from build123d import *

# Parameters (mm, degrees)
SKETCH1_W           = 40.5
SKETCH1_H           = 20
BOSS_EXTRUDE1_DEPTH = 41
SKETCH2_W           = 56.4
SKETCH2_H           = 20
SKETCH2_R           = 2.25
BOSS_EXTRUDE2_DEPTH = 3.5
SKETCH3_R           = 3
BOSS_EXTRUDE3_DEPTH = 6
SKETCH4_W           = 10
SKETCH4_H           = 3.5
BOSS_EXTRUDE4_DEPTH = 5
FILLET1_R           = 2
FILLET2_R           = 1
FILLET3_R           = 1


with BuildPart() as part:
    # Sketch1 → Boss-Extrude1 (new body)
    with BuildSketch(Plane(origin=(0, 0, 0), x_dir=(1, 0, 0), z_dir=(0, 1, 0))):
        Rectangle(SKETCH1_W, SKETCH1_H)
    extrude(amount=BOSS_EXTRUDE1_DEPTH)

    # Sketch2 → Boss-Extrude2 (add)
    with BuildSketch(Plane(origin=(0, 28, 0), x_dir=(-1, 0, 0), z_dir=(0, -1, 0))):
        Rectangle(SKETCH2_W, SKETCH2_H)
        with Locations(Location((-24, 5, 0), (0, 0, 90))):
            Circle(SKETCH2_R, mode=Mode.SUBTRACT)
        with Locations(Location((24, 5, 0), (0, 0, 90))):
            Circle(SKETCH2_R, mode=Mode.SUBTRACT)
        with Locations(Location((24, -5, 0), (0, 0, 90))):
            Circle(SKETCH2_R, mode=Mode.SUBTRACT)
        with Locations(Location((-24, -5, 0), (0, 0, 90))):
            Circle(SKETCH2_R, mode=Mode.SUBTRACT)
    extrude(amount=-BOSS_EXTRUDE2_DEPTH)

    # Sketch3 → Boss-Extrude3 (add)
    with BuildSketch(Plane(origin=(0, 41, 0), x_dir=(1, 0, 0), z_dir=(0, 1, 0))):
        with Locations(Location((-10.5, 0, 0), (0, 0, 270))):
            Circle(SKETCH3_R)
    extrude(amount=BOSS_EXTRUDE3_DEPTH)

    # Sketch4 → Boss-Extrude4 (add)
    with BuildSketch(Plane.ZY.offset(20.25)):
        with Locations((0, 5.25)):
            Rectangle(SKETCH4_W, SKETCH4_H)
    extrude(amount=BOSS_EXTRUDE4_DEPTH)

    # Fillet1
    fillet1_edges = [part.edges().sort_by_distance(p)[0] for p in [
        (28.2, 29.75, -10),
        (-28.2, 29.75, 10),
        (28.2, 29.75, 10),
        (-28.2, 29.75, -10),
    ]]
    fillet(fillet1_edges, radius=FILLET1_R)

    # Fillet2
    fillet2_edges = [part.edges().sort_by_distance(p)[0] for p in [
        (20.25, 14, 10),
        (-20.25, 14, 10),
        (-20.25, 14, -10),
        (20.25, 14, -10),
        (0, 0, 10),
        (-20.25, 0, 0),
        (0, 0, -10),
        (20.25, 0, 0),
        (-20.25, 36.25, 10),
        (-20.25, 36.25, -10),
    ]]
    fillet(fillet2_edges, radius=FILLET2_R)

    # Fillet3
    fillet3_edges = [part.edges().sort_by_distance(p)[0] for p in [
        (0.5, 41, 10),
        (-20.25, 41, 0),
        (-19.957106781, 41, 9.707106781),
        (-19.957106781, 41, -9.707106781),
        (20.25, 41, 0),
        (20.25, 36.25, 10),
        (20.25, 36.25, -10),
        (0.5, 41, -10),
    ]]
    fillet(fillet3_edges, radius=FILLET3_R)


solid = part.part
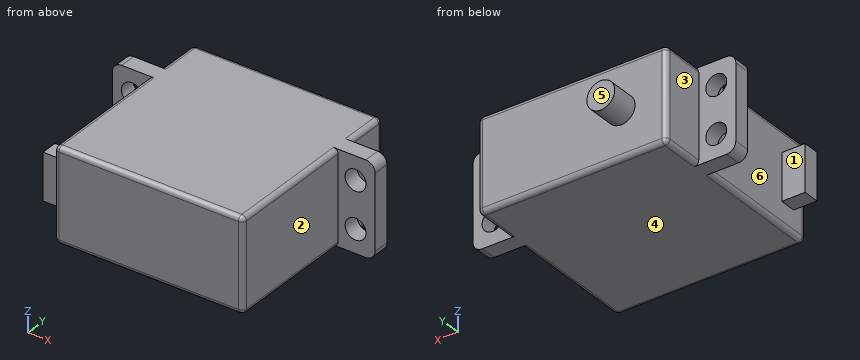
Part model, mm, in its own coordinate system. Face numbers are marked on the shaded views. A direction names the side the tool comes from. Coordinates: 2 decimals unless noted, no trailing zeros. Loops run counter-clockwise (first coordinate to the right, second up) from the corner with the lowest first, then second, coordinate; pieces in that order, holes last. Notation, with made-up numbers: (36, 53) - (47, 53) arc R29 ccw to (47, 86) - close; hole circle Ø10 at (74, 38.5). An arc over 180 degrees is marked (long way). Write each question's results on one line, items separated by ' | '. Start each with the question number.
Q1. Probe line 1 along X through (y, z) = (29.4, -5); line 2 along Y through (x, z) = (-13, -2.5); line 3 along X through (y, z) = (37, -3). List the from-to ranges inside material, lowest first.
Q2. Slice it at C-C on x = 24. Give the cut face in (y, z).
Q3. Drop flat-ended pins along their axis: pin 1 Ø2.5 at (x, z) = (-24, -5) entering from +Y; pin 2 Ø9 at (y, z) = (11, -1) entering from +X; pin 3 Ø3 at (x, y) = (-21.5, 5.5) entering from -Z; pin 4 Ø3 at (x, y) = (-22.5, 11.5) entering from +Z. Give the stop position or say it passes through.
Q4. Slice it at D-D on y = 34. Give the cut face in (x, z), and give its area (3 significant figures).
Q5. Two-plate mould, pull along Y, no slides. Class the marked faces 4, 5 and 6: +Y half, -Y half, draft (parallel to the pull), parting line (faces both ways), or undercut.
Q6. Which spindle directions (+Z, -Z, +X, -X, +Y, -Y) get a long thin tool onto all of the face, cutting with end or side? Do the marked faces 1, 2 and 3. Say none if no direction does.
Q7. Slice it at B-B on z = 0. Give the cut face in (x, y).
Q8. Slice it at A-A on x = -21. Give the cut face in (y, z), and give its area (3 significant figures).
Answer:
1) line 1: x = -28.2 to -26.25, -21.75 to 21.75, 26.25 to 28.2 | line 2: y = 0 to 41 | line 3: x = -20.25 to 20.25
2) outline: (28, -10) - (31.5, -10) - (31.5, -7.25) - (28, -7.25) - close; (28, -2.75) - (31.5, -2.75) - (31.5, 2.75) - (28, 2.75) - close; (28, 7.25) - (31.5, 7.25) - (31.5, 10) - (28, 10) - close
3) pin 1: stops at y = 7 | pin 2: stops at x = 20.25 | pin 3: stops at z = -9.66 | pin 4: passes through
4) outline: (-20.25, -9) arc R1 ccw to (-19.25, -10) - (19.25, -10) arc R1 ccw to (20.25, -9) - (20.25, 9) arc R1 ccw to (19.25, 10) - (-19.25, 10) arc R1 ccw to (-20.25, 9) - close | area: 809 mm2
5) face 4: draft | face 5: +Y half | face 6: undercut
6) face 1: +Z, -Z, -X | face 2: +Z, -Z, +X, -Y | face 3: +Z, -Z, -X, +Y
7) outline: (-28.2, 28) - (-20.25, 28) - (-20.25, 7) - (-25.25, 7) - (-25.25, 3.5) - (-20.25, 3.5) - (-20.25, 1) arc R1 ccw to (-19.25, 0) - (19.25, 0) arc R1 ccw to (20.25, 1) - (20.25, 28) - (28.2, 28) - (28.2, 31.5) - (20.25, 31.5) - (20.25, 40) arc R1 ccw to (19.25, 41) - (-7.5, 41) - (-7.5, 47) - (-13.5, 47) - (-13.5, 41) - (-19.25, 41) arc R1 ccw to (-20.25, 40) - (-20.25, 31.5) - (-28.2, 31.5) - close
8) outline: (3.5, -5) - (7, -5) - (7, 5) - (3.5, 5) - close; (28, -10) - (31.5, -10) - (31.5, 10) - (28, 10) - close | area: 105 mm2
